Geometry: see drawing. Coordinates: mm, zero at the bounding-box minimum. Round coordinates to 2 decimals unless told otherwise and drop trailing zeros. Loops run counter-clockwise (first coordinate to the right, second up) from the corner with the lowest first, then second, coordinate; pieces in that order, holes last. Notation, with made-up numbers: (-24.5, 55) -> (33.5, 55) arc R18 ccw to (33.5, 66) -> close; hole circle Ø9 at (5.25, -21.5). An arc over 180 degrees is marked (long way). Write item = value, one per line.
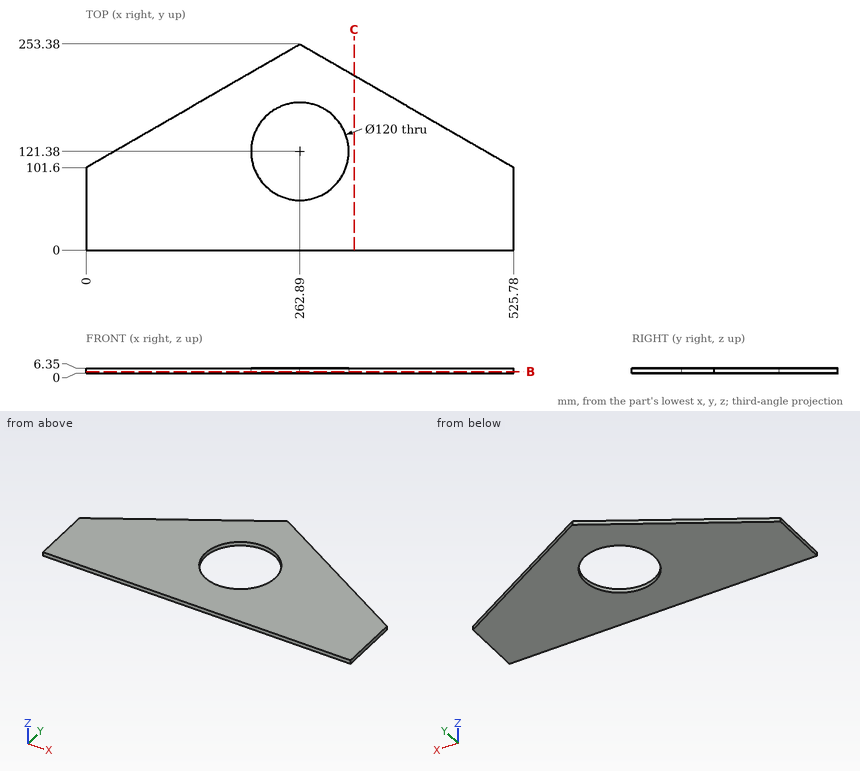
1. Section query B-B (z = 2). Return the cut outline in (x, y), then the cut area to 3 significant figures.
Evaluation:
outline = (0, 0) -> (525.78, 0) -> (525.78, 101.6) -> (262.89, 253.38) -> (0, 101.6) -> close; hole circle Ø120 at (262.89, 121.38)
area = 82,000 mm²
2. Section query C-C (x = 329.5). Return the cut outline in (y, z).
Evaluation:
outline = (0, 0) -> (214.92, 0) -> (214.92, 6.35) -> (0, 6.35) -> close
3. Line query: probe 1 along Y at (x, z) = (262.89, 3.5); probe 2 along X at (y, z) = (119, 1.5) (1 decimal); probe 3 along Y at (x, z) = (249, 5). Output: solid intervals per line, ascending. Write a range as from..to.
Evaluation:
probe_1 = 0..61.38, 181.38..253.38
probe_2 = 30.1..202.9, 322.8..495.6
probe_3 = 0..63.01, 179.75..245.36
4. Contact query for flat-ended pins moving along their axis: pin 1 Ø3 at (y, z) = (208.5, 1.5) entering from +X; pin 2 Ø1.5 at (x, z) = (236, 1.5) entering from +Y. Output: stop coordinate, or through.
Evaluation:
pin_1 = 343.22
pin_2 = 238.29
